For this review, take the finished solid that the model builds, in its own axes (mm). A direction names the side the tool comes from. Round coordinates to 2 decimals unless told otherwise and drop trailing zeros. Loops run counter-clockwise (first coordinate to the right, second up) from the corner with the lowest first, then second, coordinate; pieces in that order, holes last.
1. Tool access review of faces 4 (the flat face through (7.764, -4.553, 2.465)), 5 (the cylindrical face through (0.74, 3.32, 7.6)), 6 (the cylindrical face through (-6, 0, 16)): name each direction out of +Z, -Z, +X, -X, +Y, -Y from which nothing blocks a thin tool from reaching the whole face with its end or side.
2. Consider section A-A on z = 10. State the section outline as (x, y) points, then the cut area to 3 significant figures.
3. Consider section C-C on y = -7.5. State the section outline as (x, z) points, then the cut area to 3 significant figures.
4. Consider section B-B on z = 20. State the section outline as (x, y) points, then the cut area to 3 significant figures.
5. To check wall thickness, follow line 1 along Y through (x, z) = (0, 10.75); line 2 along Z through (x, y) = (6, 6.25); line 3 along Y through (x, z) = (2.5, 1.5). State the ranges of each line that lie inside material, in increasing order.
6. Consider section D-D on x = -6.5. State the section outline as (y, z) points.
7. Draft analysis for pull direction X (two halves, no side actions). For faces 1 (the conical face through (-0.128, 0.576, 16.688)), 2 (the flat face through (-5, 4, 5)), 3 (the flat face through (-7.764, 4.553, 2.465)), state which applies: released by +X, released by -X, zero draft, split by the parting line, or undercut.
8. Clearance check with flat-ended pins moving along their axes: pin 1 Ø10 at (y, z) = (-5, 18.5) entering from -X; pin 2 Ø6 at (y, z) = (0.5, 4) entering from -X; pin 3 Ø4 at (x, z) = (7.5, 8) entering from -Y; pin 4 Ø1.5 at (x, z) = (-0.5, 14) entering from +Y. State where each tip first meets the part, or that it passes through.
from build123d import *

# Parameters (mm, degrees)
EXTRUDE_1_DEPTH     = 5
SKETCH_2_R          = 6
EXTRUDE_2_DEPTH     = 24
M8X1_25_1_D         = 6.8
M8X1_25_1_DEPTH     = 15
M8X1_25_1_TIP       = 2.042926105
SKETCH_5_OUTSIDE_W  = 30.776
SKETCH_5_OUTSIDE_H  = 27.992
SKETCH_5_OUTSIDE_R  = 10
CUT_EXTRUDE_1_DEPTH = 28.658633372
CHAMFER_1_SIZE      = 1


with BuildPart() as part:
    # 草图1 → 凸台-拉伸1 (new body)
    with BuildSketch(Plane.XY):
        Polygon((10.392304845, 0), (5.196152423, 9), (-5.196152423, 9), (-10.392304845, 0), (-5.196152423, -9), (5.196152423, -9), align=None)
    extrude(amount=EXTRUDE_1_DEPTH)

    # 草图2 → 凸台-拉伸2 (add)
    with BuildSketch(Plane.XY.offset(5)):
        Circle(SKETCH_2_R)
    extrude(amount=EXTRUDE_2_DEPTH)

    # M8x1.25 螺纹孔1
    with Locations(Plane(origin=(-3.351254267, -2.461520779, 0), x_dir=(1, 0, 0), z_dir=(0, 0, -1))):
        with Locations((3.351254267, -2.461520779)):
            Hole(M8X1_25_1_D / 2, depth=M8X1_25_1_DEPTH)
            with Locations((0, 0, -(M8X1_25_1_DEPTH + M8X1_25_1_TIP / 2))):  # 118° drill point
                Cone(0, M8X1_25_1_D / 2, M8X1_25_1_TIP, mode=Mode.SUBTRACT)

    # 草图5 outside → 切除-拉伸1 (cut, through all)
    with BuildSketch(Plane.XY.offset(5)):
        Rectangle(SKETCH_5_OUTSIDE_W, SKETCH_5_OUTSIDE_H)
        Circle(SKETCH_5_OUTSIDE_R, mode=Mode.SUBTRACT)
    extrude(amount=-CUT_EXTRUDE_1_DEPTH, mode=Mode.SUBTRACT)

    # 倒角1
    chamfer_1_edges = [part.edges().sort_by_distance(p)[0] for p in [
        (-6, 0, 29),
    ]]
    chamfer(chamfer_1_edges, length=CHAMFER_1_SIZE)


solid = part.part
Resolved:
1. face 4: +Z, -Z, +X, -Y
1. face 5: -Z
1. face 6: +Z
2. outline: circle Ø12 at (0, 0); hole circle Ø6.8 at (0, 0)
2. area: 76.8 mm2
3. outline: (-6.06, 0) - (6.06, 0) - (6.06, 5) - (-6.06, 5) - close
3. area: 60.6 mm2
4. outline: circle Ø12 at (0, 0)
4. area: 113 mm2
5. line 1: y = -6 to -3.4, 3.4 to 6
5. line 2: z = 0 to 5
5. line 3: y = -9 to -2.3, 2.3 to 9
6. outline: (-6.74, 0) - (6.74, 0) - (6.74, 5) - (-6.74, 5) - close
7. face 1: undercut
7. face 2: zero draft
7. face 3: released by -X
8. pin 1: stops at x = -6
8. pin 2: stops at x = -10
8. pin 3: stops at y = -2.4
8. pin 4: stops at y = 6
